Could you check a few things on this model? Use its own coordinates, in mm. A direction names the side the tool comes from. Give positions to 0.01 mm unless a question says otherwise; leave off trailing zeros. Write each loop counter-clockwise with the first axis right and the second up, starting at its lowest first coordinate (ties: lowest second). Pieces come first, ordered by that corner, then holes. Notation, with made-up numbers: M 65,-38.75 L 70,-38.75 A22 ccw 70,-30.75 Z; hole C 78.5,39 d1. An arc over 180 degrees is marked long. Answer as a JSON object with one key per item and string values. Group by question number.
```python
from build123d import *

# Parameters (mm, degrees)
SKETCH2_W               = 15
SKETCH2_H               = 15
BOSS_EXTRUDE3_DEPTH     = 30
SKETCH1_R               = 2
CUT_EXTRUDE1_DEPTH      = 16
SKETCH3_W               = 4.5
SKETCH3_H               = 19
CUT_EXTRUDE2_DEPTH      = 8.5
CUT_EXTRUDE2_DEPTH_BACK = 8.5
SKETCH5_R               = 1.5
CUT_EXTRUDE3_DEPTH      = 3.6
SKETCH5_2_R             = 1.5
CUT_EXTRUDE4_DEPTH      = 31
FILLET3_R               = 3
FILLET1_R               = 1
SKETCH6_R               = 2.8
CUT_EXTRUDE5_DEPTH      = 20
CUT_EXTRUDE5_DEPTH_BACK = 3.25


with BuildPart() as part:
    # Sketch2 → Boss-Extrude3 (new body)
    with BuildSketch(Plane(origin=(0, 0, 0), x_dir=(1, 0, 0), z_dir=(0, 1, 0))):
        Rectangle(SKETCH2_W, SKETCH2_H)
    extrude(amount=BOSS_EXTRUDE3_DEPTH)

    # Sketch1 → Cut-Extrude1 (cut, through all)
    with BuildSketch(Plane.XY.offset(7.5)):
        with Locations((0, 4)):
            Circle(SKETCH1_R)
        with Locations((0, 14)):
            Circle(SKETCH1_R)
    extrude(amount=-CUT_EXTRUDE1_DEPTH, mode=Mode.SUBTRACT)

    # Sketch3 → Cut-Extrude2 (cut, two sides)
    with BuildSketch(Plane(origin=(0, 0, 0), x_dir=(0, 0, -1), z_dir=(1, 0, 0))) as cut_extrude2_sk:
        with Locations((0, 9.5)):
            Rectangle(SKETCH3_W, SKETCH3_H)
    extrude(amount=CUT_EXTRUDE2_DEPTH, mode=Mode.SUBTRACT)
    extrude(cut_extrude2_sk.sketch, amount=-CUT_EXTRUDE2_DEPTH_BACK, mode=Mode.SUBTRACT)

    # Sketch5 → Cut-Extrude3 (cut)
    with BuildSketch(Plane(origin=(0, 30, 0), x_dir=(1, 0, 0), z_dir=(0, 1, 0))):
        with BuildLine():
            Line((-2.107130751, -3.4), (2.107130751, -3.4))
            ThreePointArc((2.107130751, -3.4), (4, 0), (2.107130751, 3.4))
            Line((2.107130751, 3.4), (-2.107130751, 3.4))
            ThreePointArc((-2.107130751, 3.4), (-4, 0), (-2.107130751, -3.4))
        make_face()
        Circle(SKETCH5_R, mode=Mode.SUBTRACT)
    extrude(amount=-CUT_EXTRUDE3_DEPTH, mode=Mode.SUBTRACT)

    # Sketch5<2> → Cut-Extrude4 (cut, through all)
    with BuildSketch(Plane(origin=(0, 30, 0), x_dir=(1, 0, 0), z_dir=(0, 1, 0))):
        Circle(SKETCH5_2_R)
    extrude(amount=-CUT_EXTRUDE4_DEPTH, mode=Mode.SUBTRACT)

    # Fillet3
    fillet3_edges = [part.edges().sort_by_distance(p)[0] for p in [
        (7.5, 0, -4.875),
        (-7.5, 0, 4.875),
        (-7.5, 0, -4.875),
        (7.5, 0, 4.875),
    ]]
    fillet(fillet3_edges, radius=FILLET3_R)

    # Fillet1
    fillet1_edges = [part.edges().sort_by_distance(p)[0] for p in [
        (0, 0, -7.5),
        (6.621320344, 0.878679656, -7.5),
        (-6.621320344, 0.878679656, -7.5),
        (7.5, 16.5, 7.5),
        (-7.5, 16.5, 7.5),
        (0, 0, 7.5),
        (-7.5, 16.5, -7.5),
        (7.5, 16.5, -7.5),
        (-6.621320344, 0.878679656, 7.5),
        (6.621320344, 0.878679656, 7.5),
    ]]
    fillet(fillet1_edges, radius=FILLET1_R)

    # Sketch6 → Cut-Extrude5 (cut, two sides)
    with BuildSketch(Plane.XZ.offset(-19)) as cut_extrude5_sk:
        Circle(SKETCH6_R)
    extrude(amount=CUT_EXTRUDE5_DEPTH, mode=Mode.SUBTRACT)
    extrude(cut_extrude5_sk.sketch, amount=-CUT_EXTRUDE5_DEPTH_BACK, mode=Mode.SUBTRACT)


solid = part.part
```
1) Please list where these lines run through material, in increasing order: line 1 along Y through (x, z) = (0, 5.5); line 2 along Z through (x, y) = (2, 16); line 3 along X through (y, z) = (4, -4.5). Write a range as from..to.
2) If we section it at D-D, the plane y = 27: List the corners of the cut face in (x, z) for me, plus the area to 3 significant figures.
3) We'd pull the mould along Y, two halves only. Please class faces 1 (the cylindrical face through (-2, 4, 5)), 2 (the cylindrical face through (6.6, 0.86, -4.4)), 3 (the flat face through (0, 26.4, -2)): released by +Y, released by -Y, zero draft, split by the parting line, or undercut.
4) If we section it at B-B, the plane z = -3.75: List the corners of the cut face in (x, y) for me, plus the area to 3 significant figures.
5) I'm going to push flat-ended pins straight in: pin 1 (6 mm diameter, centred on x = 0.5, z = 2, fed in from -Y); pin 2 (1.3 mm diameter, centred on x = -3, z = 0, fed in from -Y); pin 3 (1 mm diameter, centred on y = 12.5, z = -1.5, fed in from +X); pin 4 (5.5 mm diameter, centred on x = 0, z = 0.5, fed in from +Y). Where does each tip first touch, or does it pass through?
6) If we section it at C-C, the plane x = 0: Give the number of separate pieces and of enclosed holes in the cut face, plus the area to 3 significant figures.
7) For faces 4 (the flat face through (5, 9, 2.25)), 5 (the flat face through (0, 28, -3.4)), 6 (the cylindrical face through (0, 1.1, -2.8)), which set-ups out of +Z, -Z, +X, -X, +Y, -Y let a thin tool reach every point of the face, with its end or its side?
8) If we section it at A-A, the plane y = 10: List the corners of the cut face in (x, z) for me.
Taken from the geometry:
{
 "1": {"line 1": "0..2, 6..12, 16..30", "line 2": "-7.5..-2.25, 2.25..7.5", "line 3": "-7.5..-2, 2..7.5"},
 "2": {"outline": "M -7.5,-6.5 A1 ccw -6.5,-7.5 L 6.5,-7.5 A1 ccw 7.5,-6.5 L 7.5,6.5 A1 ccw 6.5,7.5 L -6.5,7.5 A1 ccw -7.5,6.5 Z; hole M -2.11,-3.4 L 2.11,-3.4 A4 ccw 2.11,3.4 L -2.11,3.4 A4 ccw Z", "area": "177 mm²"},
 "3": {"face 1": "undercut", "face 2": "released by -Y", "face 3": "released by +Y"},
 "4": {"outline": "M -7.5,3 A3 ccw -4.5,0 L 4.5,0 A3 ccw 7.5,3 L 7.5,30 L -7.5,30 Z; hole C 0,4 d4; hole C 0,14 d4", "area": "421 mm²"},
 "5": {"pin 1": "y = 0", "pin 2": "y = 19", "pin 3": "through", "pin 4": "y = 26.4"},
 "6": {"separate pieces": "6", "enclosed holes": "0", "area": "213 mm²"},
 "7": {"face 4": "+X, -X, -Y", "face 5": "+Y", "face 6": "-Y"},
 "8": {"outline": "M -7.5,-6.5 A1 ccw -6.5,-7.5 L 6.5,-7.5 A1 ccw 7.5,-6.5 L 7.5,-2.25 L 1.67,-2.25 A2.8 cw -1.67,-2.25 L -7.5,-2.25 Z; M -7.5,2.25 L -1.67,2.25 A2.8 cw 1.67,2.25 L 7.5,2.25 L 7.5,6.5 A1 ccw 6.5,7.5 L -6.5,7.5 A1 ccw -7.5,6.5 Z"}
}
